Can you work these out from the drawing? Everything is in mm from the part's minimum corner. Round coordinates to 2 decimals unless told otherwise and drop trailing zeros. Loops run counter-clockwise (first coordinate to the right, second up) from the corner with the lowest first, then second, coordinate; pieces in that order, holes last. Notation, with made-up numbers: (47, 78) - (60, 78) arc R27 ccw to (60, 95) - close; hole circle Ø9 at (-11.5, -29.75). An arc over 180 degrees is marked (long way). Answer as CSV lines item,"result". Start each with the question number.
1) I'm going to push flat-ended pins straight in: pin 1 Ø8 at (x, z) = (13, 32.5) entering from +Y; pin 2 Ø3 at (x, y) = (32.5, 4.5) entering from -Z. Where does each tip first touch, or does it pass through?
2) We'd pull the mould along X, two halves only. Please class the marked faces 1, 2 and 3: pulls with the +X half, pulls with the -X half, needs draft (parallel to the pull), parting line crosses it, or undercut.
3) Please list where these lines run through material, in increasing order: line 1 along Y through (x, z) = (1, 54); line 2 along X through (y, z) = (2.1, 21); line 3 along Y through (x, z) = (13, 38).
4) Suppose I cut it at A-A, the plane z = 54. Write out the boundary of the cut face in (x, y).
5) Suppose I cut it at B-B, the plane y = 4. Write out the boundary of the cut face in (x, z), then the cut area to 3 significant figures.
6) Suppose I cut it at C-C, the plane x = 8.5. Write out the boundary of the cut face in (y, z).
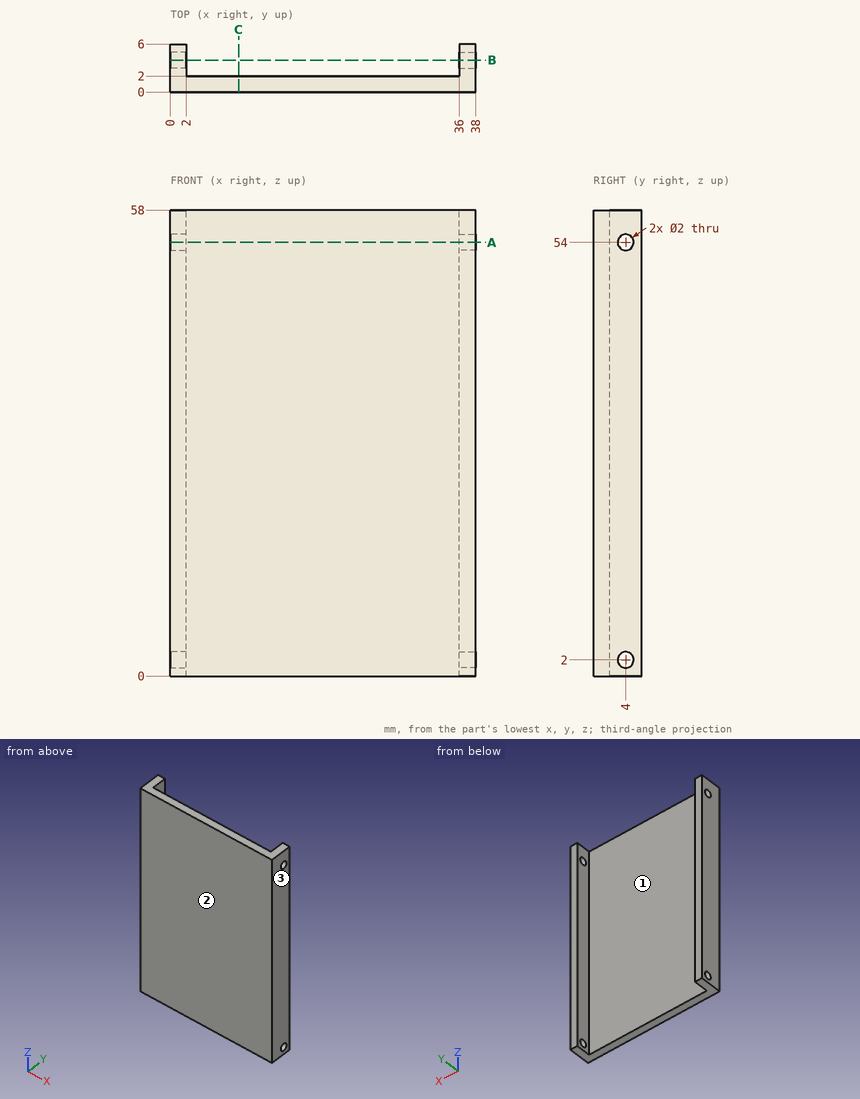
Filled sheet:
1,pin 1,"y = 2"
1,pin 2,"through"
2,face 1,"undercut"
2,face 2,"needs draft"
2,face 3,"pulls with the +X half"
3,line 1,"0 to 3, 5 to 6"
3,line 2,"0 to 2, 36 to 38"
3,line 3,"0 to 2"
4,outline,"(0, 0) - (38, 0) - (38, 3) - (36, 3) - (36, 2) - (2, 2) - (2, 3) - (0, 3) - close; (0, 5) - (2, 5) - (2, 6) - (0, 6) - close; (36, 5) - (38, 5) - (38, 6) - (36, 6) - close"
5,outline,"(0, 0) - (2, 0) - (2, 1) - (0, 1) - close; (0, 3) - (2, 3) - (2, 53) - (0, 53) - close; (0, 55) - (2, 55) - (2, 58) - (0, 58) - close; (36, 0) - (38, 0) - (38, 1) - (36, 1) - close; (36, 3) - (38, 3) - (38, 53) - (36, 53) - close; (36, 55) - (38, 55) - (38, 58) - (36, 58) - close"
5,area,"216 mm²"
6,outline,"(0, 0) - (2, 0) - (2, 58) - (0, 58) - close"
